For this review, take the finished solid that the model builds, in its own axes (mm). Face numbers are marked on the shaded views. Coordinates: 2 decimals unless noted, no trailing zeros. Loops run counter-clockwise (first coordinate to the right, second up) from the corner with the lowest first, then second, coordinate; pieces in that order, holes last. Notation, with made-up numbers: (30.5, -37) -> (83.5, -37) arc R16 cw to (83.5, -14) -> close; hole circle Ø7 at (46.25, 52). An arc over 180 degrees is marked (long way). Use a Markdown table: item, result.
from build123d import *


with BuildPart() as part:
    # Эскиз1 → Повернуть2 (revolve)
    with BuildSketch(Plane(origin=(0, 0, 0), x_dir=(0, 0, -1), z_dir=(1, 0, 0))):
        Polygon((0, 8.5), (188.5, 8.5), (188.5, 67.5), (192.5, 67.5), (192.5, 52), (211, 52), (211, 0), (0, 0), align=None)
    revolve_2 = revolve(axis=Axis((0, 0, 0), (0, 0, -1)))

    # Зеркальное отражение1: Повернуть2 across plane
    add(revolve_2.mirror(Plane(origin=(0, 8.5, 0), x_dir=(1, 0, 0), z_dir=(0, 0, -1))))


solid = part.part
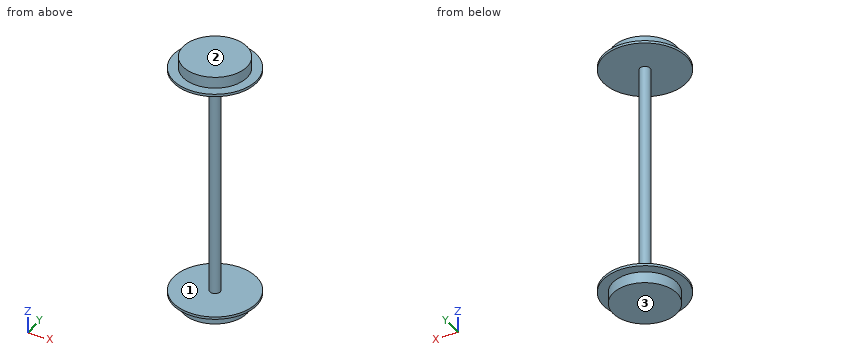
(1) Take a section at A-A on x = -22. Write out the cut boundary in (y, z), plus the area to 3 significant figures.
Found:
| item | result |
|---|---|
| outline | (-63.81, -192.5) -> (-47.12, -192.5) -> (-47.12, -211) -> (47.12, -211) -> (47.12, -192.5) -> (63.81, -192.5) -> (63.81, -188.5) -> (-63.81, -188.5) -> close; (-63.81, 188.5) -> (63.81, 188.5) -> (63.81, 192.5) -> (47.12, 192.5) -> (47.12, 211) -> (-47.12, 211) -> (-47.12, 192.5) -> (-63.81, 192.5) -> close |
| area | 4,510 mm^2 |
(2) Take a section at C-C on y = 0. Write out the cut boundary in (x, z), plus the area to 3 significant figures.
Found:
| item | result |
|---|---|
| outline | (-67.5, -192.5) -> (-52, -192.5) -> (-52, -211) -> (52, -211) -> (52, -192.5) -> (67.5, -192.5) -> (67.5, -188.5) -> (8.5, -188.5) -> (8.5, 188.5) -> (67.5, 188.5) -> (67.5, 192.5) -> (52, 192.5) -> (52, 211) -> (-52, 211) -> (-52, 192.5) -> (-67.5, 192.5) -> (-67.5, 188.5) -> (-8.5, 188.5) -> (-8.5, -188.5) -> (-67.5, -188.5) -> close |
| area | 11,300 mm^2 |
(3) Mouldability with a two-part tool opening along Z and no side actions: class the marked faces 1, 2 and 3 as pulls with the +Z half, pulls with the -Z half, needs draft (parallel to the pull), parting line crosses it, or undercut.
Found:
| item | result |
|---|---|
| face 1 | undercut |
| face 2 | pulls with the +Z half |
| face 3 | pulls with the -Z half |
(4) For line 1 along Z through (x, y) = (12.5, 56.5); line 2 along Z through (x, y) = (8, 13.5); line 3 along Y through (x, z) = (-1, 52), list the stretches that pass through material, from the lowest coordinate up.
Found:
| item | result |
|---|---|
| line 1 | z = -192.5 to -188.5, 188.5 to 192.5 |
| line 2 | z = -211 to -188.5, 188.5 to 211 |
| line 3 | y = -8.44 to 8.44 |
(5) Take a section at B-B on y = -37. Write out the cut boundary in (x, z), plus the area to 3 significant figures.
Found:
| item | result |
|---|---|
| outline | (-56.46, -192.5) -> (-36.54, -192.5) -> (-36.54, -211) -> (36.54, -211) -> (36.54, -192.5) -> (56.46, -192.5) -> (56.46, -188.5) -> (-56.46, -188.5) -> close; (-56.46, 188.5) -> (56.46, 188.5) -> (56.46, 192.5) -> (36.54, 192.5) -> (36.54, 211) -> (-36.54, 211) -> (-36.54, 192.5) -> (-56.46, 192.5) -> close |
| area | 3,610 mm^2 |
(6) For pin 1 Ø12 at (x, z) = (-9, -96) entering from +Y; pin 2 Ø6 at (x, z) = (9, 57) entering from -Y, all flat-tipped, find the tip position at first contact; note any pin that passes through.
Found:
| item | result |
|---|---|
| pin 1 | stops at y = 7.95 |
| pin 2 | stops at y = -6.02 |
